Check sheet for the modelled part. Datum: model origin and axes. Units: mm. A direction names the side the tool comes from. Round coordinates to 2 decimals unless told otherwise and drop trailing zeros. Order: outer loops, then holes, each group sorted by start corner. A loop starts at its lowest first (then second) coordinate and runs counter-clockwise, first axis right, second up. Notation, with made-up numbers: M -20,-16.5 L 28,-16.5 A22 ccw 28,5.5 Z; hole C 19,72 d11. An arc over 180 degrees is marked long. One line per item, written item: value. Start each with the question number.
(1) Depth check by flat-ended pin: pin 1 Ø3 at (y, z) = (0.5, 19.5) entering from +X; pin 2 Ø11 at (x, z) = (-14, 21) entering from +Y; pin 3 Ø15 at (y, z) = (-4.5, 18.5) entering from -X. Enter the tip coordinate at first touch or a pass-through.
(2) Cross-section at A-A, the plane y = -19.5. Enter the section's corners in (x, z), and give its area (3 significant figures).
(3) Cross-section at C-C, the plane x = 14. Enter the section's corners in (y, z).
(4) Cross-section at B-B, the plane z = 14. Enter the section's corners in (x, y), and give its area (3 significant figures).
(5) Cross-section at D-D, the plane y = -5. Enter the section's corners in (x, z), and give its area (3 significant figures).
(6) Thickness scan on L1, parallel to X at y = -19.5, z = 18.75; L2, parallel to Y at x = -7, z = 13.5; L3, parallel to Y at x = -9.5, z = 11.75. Record the ranges inside material, lowest first.
(7) Release check for a two-part mould opening along X. For faces 6 (the face through (31.958, -23, 15)), 7 (the face through (7, -3, 0)), 8 (the face through (-18.042, -23, 15)), 9 (the face through (7, -17.406, 15)) record: released by +X, released by -X, zero draft, split by the parting line, or undercut.
(8) Access from +Z, -Z, +X, -X, +Y, -Y to the whole of each face (thin tool, end or side, straight path). Record for faces 1 (the face through (7, 15.594, 15)), 2 (the face through (27, -14.406, 15)), 3 (the face through (-15.042, -25, 15)), 4 (the face through (7, -3, 30)), 5 (the face through (-13, -14.406, 15)).
from build123d import *

# Parameters (mm, degrees)
SKETCH_1_W          = 30
SKETCH_1_H          = 30
EXTRUDE_1_DEPTH     = 30
SKETCH_2_W          = 50
SKETCH_2_H          = 40
EXTRUDE_2_DEPTH     = 3
SKETCH_3_W          = 3
SKETCH_3_H          = 40
EXTRUDE_3_DEPTH     = 15
SKETCH_4_W          = 50.744831967
SKETCH_4_H          = 10
CUT_EXTRUDE_1_DEPTH = 19


with BuildPart() as part:
    # 草图1 → 凸台-拉伸1 (new body)
    with BuildSketch(Plane.XY):
        with Locations((6.958041958, 0.594405594)):
            Rectangle(SKETCH_1_W, SKETCH_1_H)
    extrude(amount=EXTRUDE_1_DEPTH)

    # 草图2 → 凸台-拉伸2 (add)
    with BuildSketch(Plane.XZ.offset(14.405594406)):
        with Locations((6.958041958, 20)):
            Rectangle(SKETCH_2_W, SKETCH_2_H)
    extrude(amount=EXTRUDE_2_DEPTH)

    # 草图3 → 凸台-拉伸3 (add)
    with BuildSketch(Plane.XZ.offset(17.405594406)):
        with Locations((-16.541958042, 20)):
            Rectangle(SKETCH_3_W, SKETCH_3_H)
        with Locations((30.458041958, 20)):
            Rectangle(SKETCH_3_W, SKETCH_3_H)
    extrude(amount=EXTRUDE_3_DEPTH)

    # 草图4 → 切除-拉伸1 (cut, through all)
    with BuildSketch(Plane(origin=(0, -14.405594406, 0), x_dir=(1, 0, 0), z_dir=(0, 1, 0))):
        with Locations((6.585625975, -35)):
            Rectangle(SKETCH_4_W, SKETCH_4_H)
    extrude(amount=-CUT_EXTRUDE_1_DEPTH, mode=Mode.SUBTRACT)


solid = part.part
Values found:
1. pin 1: x = 21.96
1. pin 2: y = -14.41
1. pin 3: x = -8.04
2. outline: M -18.04,0 L -15.04,0 L -15.04,30 L -18.04,30 Z; M 28.96,0 L 31.96,0 L 31.96,30 L 28.96,30 Z
2. area: 180 mm^2
3. outline: M -17.41,0 L 15.59,0 L 15.59,30 L -17.41,30 Z
4. outline: M -18.04,-32.41 L -15.04,-32.41 L -15.04,-17.41 L 28.96,-17.41 L 28.96,-32.41 L 31.96,-32.41 L 31.96,-14.41 L 21.96,-14.41 L 21.96,15.59 L -8.04,15.59 L -8.04,-14.41 L -18.04,-14.41 Z
4. area: 1,140 mm^2
5. outline: M -8.04,0 L 21.96,0 L 21.96,30 L -8.04,30 Z
5. area: 900 mm^2
6. L1: -18.04 to -15.04, 28.96 to 31.96
6. L2: -17.41 to 15.59
6. L3: -17.41 to -14.41
7. face 6: released by +X
7. face 7: zero draft
7. face 8: released by -X
7. face 9: undercut
8. face 1: +Z, -Z, +X, -X, +Y
8. face 2: +Z, -Z, +X, +Y
8. face 3: +Z, -Z, -Y
8. face 4: +Z, +X, -X, +Y, -Y
8. face 5: +Z, -Z, -X, +Y
